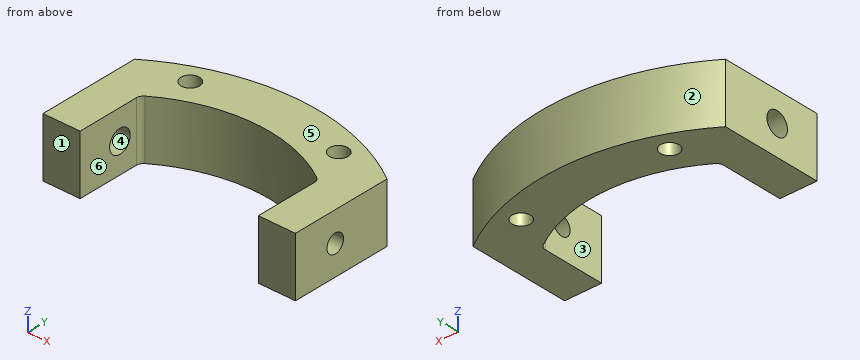
```python
from build123d import *

# Parameters (mm, degrees)
SKETCH_4_R          = 1.25
EXTRUDE_2_DEPTH     = 8
SKETCH_5_W          = 4.5
SKETCH_5_H          = 18.121653049
CUT_EXTRUDE_2_DEPTH = 9
SKETCH_6_R          = 1.25
CUT_EXTRUDE_3_DEPTH = 35
SKETCH_7_R          = 1.55
CUT_EXTRUDE_4_DEPTH = 6
FILLET_1_R          = 1


with BuildPart() as part:
    # 草图4 → 凸台-拉伸2 (new body)
    with BuildSketch(Plane.XY):
        with BuildLine():
            Line((-21.5, 5), (-21.5, -5))
            Line((-21.5, -5), (21.5, -5))
            Line((21.5, -5), (21.5, 5))
            ThreePointArc((21.5, 5), (0, 14.077524047), (-21.5, 5))
        make_face()
        with Locations((-10, 9.361795295)):
            Circle(SKETCH_4_R, mode=Mode.SUBTRACT)
        with Locations((10, 9.361795295)):
            Circle(SKETCH_4_R, mode=Mode.SUBTRACT)
    extrude(amount=EXTRUDE_2_DEPTH)

    # 草图5 → 切除-拉伸2 (cut, through all)
    with BuildSketch(Plane.XY.offset(8)):
        with BuildLine():
            Line((-12, 4), (-12, -5))
            Line((-12, -5), (12, -5))
            Line((12, -5), (12, 4))
            ThreePointArc((12, 4), (0, 7.76631206), (-12, 4))
        make_face()
        with Locations((19.25, 4.060826525)):
            Rectangle(SKETCH_5_W, SKETCH_5_H)
        with Locations((-19.25, 4.060826525)):
            Rectangle(SKETCH_5_W, SKETCH_5_H)
    extrude(amount=-CUT_EXTRUDE_2_DEPTH, mode=Mode.SUBTRACT)

    # 草图6 → 切除-拉伸3 (cut, through all)
    with BuildSketch(Plane.ZY.offset(17)):
        with Locations((4, 1)):
            Circle(SKETCH_6_R)
    extrude(amount=-CUT_EXTRUDE_3_DEPTH, mode=Mode.SUBTRACT)

    # 草图7 → 切除-拉伸4 (cut)
    with BuildSketch(Plane.ZY.offset(17)):
        with Locations((4, 1)):
            Circle(SKETCH_7_R)
    extrude(amount=-CUT_EXTRUDE_4_DEPTH, mode=Mode.SUBTRACT)

    # 圆角1
    fillet_1_edges = [part.edges().sort_by_distance(p)[0] for p in [
        (12, 4, 4),
        (-12, 4, 4),
    ]]
    fillet(fillet_1_edges, radius=FILLET_1_R)


solid = part.part
```
CAD build for the part. Positions are in the model's coordinates, mm. Face numbers are marked on the shaded views. A direction names the side the tool comes from. Round coordinates to 2 decimals unless told otherwise and drop trailing zeros. Write each loop counter-clockwise with the first axis right and the second up, starting at its lowest first coordinate (ties: lowest second). Pieces come first, ordered by that corner, then holes. Notation, with made-up numbers: M -5.75,-25.5 L 32.25,-25.5 A21 ccw 32.25,-12.5 Z; hole C 71.25,0.25 d3. An arc over 180 degrees is marked long. One line per question, with ' | ' between items.
1. Cut at D-D on x = -10. Write the cut outline in (y, z), and give its area (3 significant figures).
Working result:
outline: M 5.23,0 L 8.11,0 L 8.11,8 L 5.23,8 Z; M 10.61,0 L 12.36,0 L 12.36,8 L 10.61,8 Z | area: 37.0 mm2
2. Probe L1, parallel to X at y = 0, z = 7.5; L2, parallel to X at y = 9, z = 3.75; L3, parallel to X at y = 9.5, z = 0.75. List the from-to ranges inside material, lowest first. Write a range as from..to.
Working result:
L1: -17..-12, 12..17 | L2: -16.7..-11.2, -8.8..8.8, 11.2..16.7 | L3: -15.93..-11.24, -8.76..8.76, 11.24..15.93
3. Cut at A-A on y = 1. Write the cut outline in (x, z), and give its area (3 significant figures).
Working result:
outline: M -17,0 L -12,0 L -12,2.45 L -17,2.45 Z; M -17,5.55 L -12,5.55 L -12,8 L -17,8 Z; M 12,0 L 17,0 L 17,2.75 L 12,2.75 Z; M 12,5.25 L 17,5.25 L 17,8 L 12,8 Z | area: 52.0 mm2
4. Mould opens along X. For the marked faces 1, 2 and 3 say: pulls with the +X half, pulls with the -X half, needs draft (parallel to the pull), parting line crosses it, or undercut.
Working result:
face 1: needs draft | face 2: parting line crosses it | face 3: undercut
5. Cut at C-C on y = -2. Write the cut outline in (x, z), and give its area (3 significant figures).
Working result:
outline: M -17,0 L -12,0 L -12,8 L -17,8 Z; M 12,0 L 17,0 L 17,8 L 12,8 Z | area: 80.0 mm2
6. Cut at B-B on z = 3.75. Write the cut outline in (x, y), and give its area (3 significant figures).
Working result:
outline: M -17,-5 L -12,-5 L -12,-0.53 L -17,-0.53 Z; M -17,2.53 L -12,2.53 L -12,3.47 A1 cw -11.55,4.3 A21 cw 11.55,4.3 A1 cw 12,3.47 L 12,2.22 L 17,2.22 L 17,8.8 A30 ccw -17,8.8 Z; M 12,-5 L 17,-5 L 17,-0.22 L 12,-0.22 Z; hole C -10,9.36 d2.5; hole C 10,9.36 d2.5 | area: 276 mm2
7. Pin check, flat tips, straight feed: pin 1 Ø4 at (x, z) = (-6.5, 4.5) entering from -Y; pin 2 Ø3 at (y, z) = (1, 4) entering from -X. Stop position of each tip, or through.
Working result:
pin 1: y = 5.97 | pin 2: x = 12
8. Which spindle directions (+Z, -Z, +X, -X, +Y, -Y) get a long thin tool onto all of the face, cutting with end or side? Do the marked faces 4, 5 and 6. Say none if no direction does.
Working result:
face 4: -X | face 5: +Z, +X, -X, +Y, -Y | face 6: +Z, -Z, -Y
